Geometry check sheet. Reference: the model listing, model coordinates, mm. A direction names the side the tool comes from. Coordinates: 2 decimals unless noted, no trailing zeros. Order: outer loops, then holes, each group sorted by start corner. A loop starts at its lowest first (then second) coordinate and runs counter-clockwise, first axis right, second up. Notation, with made-up numbers: (-0.5, -17) - (31.5, -17) arc R27 ccw to (31.5, 15) - close; hole circle Ø10 at (79, 84.25). An arc over 180 degrees is marked (long way). Return JSON: item names as keys, results as strings. Group by question number.
Item 1: Scan lines: probe 1 along Y at (x, z) = (586.5, 0.2); probe 2 along X at (y, z) = (479.5, 0.45); probe 3 along Y at (x, z) = (589.5, 0.55). Record each from-to range of solid material in increasing order.
Item 2: Draft check along Y on faces 4 (the flat face through (605.906, 499.531, 0.74)), 5 (the flat face through (580.996, 474, 1)), 6 (the flat face through (589.44, 463.6, 0.74)), 7 (the flat face through (592, 472, 0)). Enter one of: pulls with the +Y half, pulls with the -Y half, needs draft (parallel to the pull), parting line crosses it, or undercut.
Item 3: Section check D-D on z = 0.55. Give the number of separate pieces and of enclosed holes in the cut face, then the cut area to 3 significant figures.
Item 4: Tool access check on faces 1 (the cylindrical face through (602.035, 495.992, 0.74)), 2 (the flat face through (601.078, 463.645, 0.74)), 3 (the flat face through (612.32, 452.25, 0.74)). Record the directions out of +Z, -Z, +X, -X, +Y, -Y that give a thin tool (end or side, any length) a straight path to the whole face; none if there is none.
Item 5: Section check B-B on y = 471.5. Enter the section's corners in (x, z).
Item 6: Section check A-A on x = 594.5. Enter the section's corners in (y, z), then the cut area to 3 significant figures.
Item 7: Gauge pin test, flat ends, axial feed: pin 1 (0.8 mm diameter, centred on y = 453.5, z = 0.5, fed in from +X); pin 2 (2 mm diameter, centred on x = 611.34, y = 448.67, fed in from +Z) (3 decimals); pin 3 (0.8 mm diameter, centred on x = 572, z = 1, fed in from +Y). Record the tip position at first contact, or that the pin passes through.
Item 8: Section check C-C on x = 571. Enter the section's corners in (y, z).
from build123d import *

# Parameters (mm, degrees)
MODEL_R         = 1.25
EXTRUDE_1_DEPTH = 1.5


with BuildPart() as part:
    # Model → 凸台-拉伸1 (new body)
    with BuildSketch(Plane.XY):
        with BuildLine():
            Line((580.995568625, 495.770292788), (600.902512418, 495.770292788))
            ThreePointArc((600.902512418, 495.770292788), (602.050562715, 495.99865419), (603.023832761, 496.648972444))
            Line((603.023832761, 496.648972444), (608.87002472, 502.495166354))
            ThreePointArc((608.87002472, 502.495166354), (614.034668548, 502.25974311), (613.330350777, 497.137936158))
            Line((613.330350777, 497.137936158), (611.344894179, 495.770295165))
            Line((611.344894179, 495.770295165), (611.344903066, 493.770295165))
            Line((611.344903066, 493.770295165), (611.344898622, 490.139940091))
            Line((611.344898622, 490.139940091), (609.344898622, 490.139940091))
            Line((609.344898622, 490.139940091), (609.344898622, 459.003527023))
            Line((609.344898622, 459.003527023), (611.344898622, 459.003527023))
            Line((611.344898622, 459.003527023), (611.344903066, 454.922529401))
            Line((611.344903066, 454.922529401), (611.344903066, 452.922529401))
            Line((611.344903066, 452.922529401), (613.330355459, 451.554880428))
            ThreePointArc((613.330355459, 451.554880428), (614.034666789, 446.433074588), (608.870024851, 446.197653326))
            Line((608.870024851, 446.197653326), (607.649614702, 447.394418416))
            Line((607.649614702, 447.394418416), (603.130826548, 451.825656479))
            ThreePointArc((603.130826548, 451.825656479), (602.127647934, 452.488182187), (600.942551931, 452.690308661))
            Line((600.942551931, 452.690308661), (580.995568625, 452.245019157))
            Line((580.995568625, 452.245019157), (561.000550217, 451.798657335))
            Line((561.000550217, 451.798657335), (561.000550217, 456.798657335))
            Line((561.000550217, 456.798657335), (577.763165347, 455.496180974))
            ThreePointArc((577.763165347, 455.496180974), (580.033065884, 456.285210752), (580.995568625, 458.487165547))
            Line((580.995568625, 458.487165547), (580.995568625, 489.455330101))
            ThreePointArc((580.995568625, 489.455330101), (580.008584587, 491.679687702), (577.697057468, 492.440441672))
            Line((577.697057468, 492.440441672), (560.995568625, 490.770292788))
            Line((560.995568625, 490.770292788), (560.995568625, 495.100850038))
            Line((560.995568625, 495.100850038), (562.062443854, 495.770292788))
            Line((562.062443854, 495.770292788), (580.995568625, 495.770292788))
        make_face()
        with Locations((611.344898622, 500.020292788)):
            Circle(MODEL_R, mode=Mode.SUBTRACT)
        with Locations((611.344898622, 448.672527023)):
            Circle(MODEL_R, mode=Mode.SUBTRACT)
        with BuildLine():
            Line((585.91647506, 489.426366255), (604.267397119, 489.857372067))
            Line((604.267397119, 489.857372067), (597.532531309, 479.99996659))
            ThreePointArc((597.532531309, 479.99996659), (595.079201685, 478.692455827), (592.605499439, 479.961001386))
            Line((592.605499439, 479.961001386), (585.91647506, 489.426366255))
        make_face(mode=Mode.SUBTRACT)
        with BuildLine():
            Line((586.047448792, 458.632826912), (604.397047311, 458.951765009))
            Line((604.397047311, 458.951765009), (597.664323818, 468.47211859))
            ThreePointArc((597.664323818, 468.47211859), (595.190191772, 469.739825644), (592.737305457, 468.431483456))
            Line((592.737305457, 468.431483456), (586.047448792, 458.632826912))
        make_face(mode=Mode.SUBTRACT)
        with BuildLine():
            Line((583.99514789, 460.649796595), (583.995526777, 487.427452126))
            Line((583.995526777, 487.427452126), (592.089795546, 475.957499013))
            ThreePointArc((592.089795546, 475.957499013), (592.638587507, 474.250490234), (592.115726369, 472.535361137))
            Line((592.115726369, 472.535361137), (583.99514789, 460.649796595))
        make_face(mode=Mode.SUBTRACT)
        with BuildLine():
            Line((606.345062591, 460.933766521), (606.346502303, 487.858246923))
            Line((606.346502303, 487.858246923), (598.164147844, 475.898832518))
            ThreePointArc((598.164147844, 475.898832518), (597.640194793, 474.182081738), (598.190130861, 472.473476938))
            Line((598.190130861, 472.473476938), (606.345062591, 460.933766521))
        make_face(mode=Mode.SUBTRACT)
    extrude(amount=EXTRUDE_1_DEPTH)


solid = part.part
Computed:
{
 "1": {"probe 1": "y = 452.37 to 458.64, 459.3 to 464.32, 483.88 to 488.6, 489.44 to 495.77", "probe 2": "x = 581 to 584, 589.59 to 593.01, 597.1 to 600.63, 606.35 to 609.34", "probe 3": "y = 452.43 to 458.69, 463.69 to 468.71, 479.63 to 484.36, 489.51 to 495.77"},
 "2": {"face 4": "pulls with the +Y half", "face 5": "undercut", "face 6": "undercut", "face 7": "needs draft"},
 "3": {"separate pieces": "1", "enclosed holes": "6", "area": "1,040 mm²"},
 "4": {"face 1": "+Z, -Z, -X, +Y", "face 2": "+Z, -Z", "face 3": "+Z, -Z, +X"},
 "5": {"outline": "(581, 0) - (584, 0) - (584, 1.5) - (581, 1.5) - close; (591.41, 0) - (598.88, 0) - (598.88, 1.5) - (591.41, 1.5) - close; (606.35, 0) - (609.34, 0) - (609.34, 1.5) - (606.35, 1.5) - close"},
 "6": {"outline": "(452.55, 0) - (458.78, 0) - (458.78, 1.5) - (452.55, 1.5) - close; (469.65, 0) - (478.74, 0) - (478.74, 1.5) - (469.65, 1.5) - close; (489.63, 0) - (495.77, 0) - (495.77, 1.5) - (489.63, 1.5) - close", "area": "32.2 mm²"},
 "7": {"pin 1": "stops at x = 611.34", "pin 2": "passes through", "pin 3": "stops at y = 495.77"},
 "8": {"outline": "(452.02, 0) - (456.02, 0) - (456.02, 1.5) - (452.02, 1.5) - close; (491.77, 0) - (495.77, 0) - (495.77, 1.5) - (491.77, 1.5) - close"}
}
